Answer from the drawing. Dimensions are ordinates in mm from the lowest x, y and z of the part. A direction names the side the tool comes from. Coordinates: 2 decimals unless noted, no trailing zeros. Order: outer loops, then holes, each group sorted by start corner. A loop starts at its lowest first (then second) coordinate and runs counter-clockwise, first axis right, second up. Notation, with made-up numbers: (1, -27) -> (34, -27) arc R25 ccw to (34, -7) -> close; hole circle Ø4 at (-16.75, 20). An arc over 180 degrees is marked (long way). Answer as a JSON object with one key per item and string values. Group by question number.
1) Section D-D on y = 28 is taken. Determine the outline of the cut face in (x, z), and give its area (3 significant figures).
2) Determine the mould class of the marked faces 3, 4, 5 and 6 for opening direction X: released by +X, released by -X, zero draft, split by the parting line, or undercut.
3) Consider L1, parallel to Y at x = 43, z = 15.5; L2, parallel to X at y = 19.5, z = 13.75; L3, parallel to Z at x = 77.5, y = 32. Determine where each line is inside the solid, lowest interval first.
4) Section B-B on y = 4.5 is taken. Determine the outline of the cut face in (x, z).
5) Section A-A on x = 40 is taken. Determine the outline of the cut face in (y, z).
6) A tool of negligible diameter and unlimited length cuts with its end or side. For the marked faces 1 and 2, from which of +Z, -Z, +X, -X, +Y, -Y can it reach the whole face along a straight path? Write none if from no direction.
7) Section C-C on z = 5.25 is taken. Determine the outline of the cut face in (x, y), and give its area (3 significant figures).
8) Given pin 1 (2 mm diameter, centred on x = 70.5, z = 20.5, fed in from -Y), flat-ended and moving along its own axis, determine where the tip first touches the part or whether it passes through.
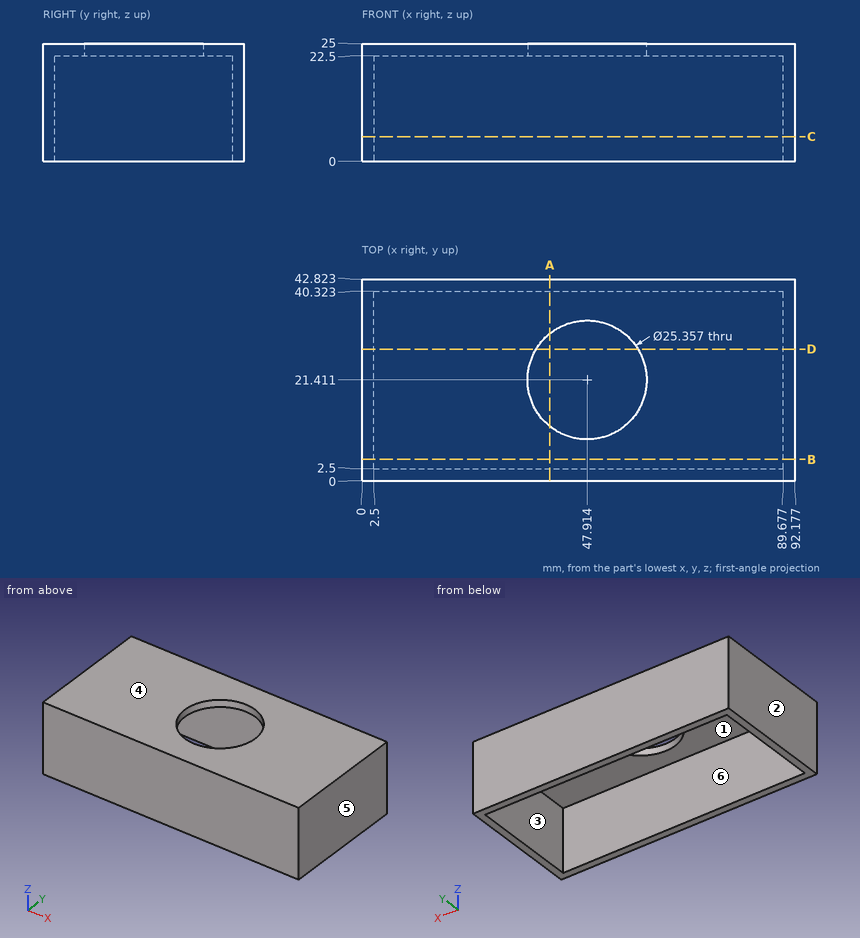
Worked answers:
{
 "1": {"outline": "(0, 0) -> (2.5, 0) -> (2.5, 22.5) -> (37.08, 22.5) -> (37.08, 25) -> (0, 25) -> close; (58.75, 22.5) -> (89.68, 22.5) -> (89.68, 0) -> (92.18, 0) -> (92.18, 25) -> (58.75, 25) -> close", "area": "289 mm²"},
 "2": {"face 3": "undercut", "face 4": "zero draft", "face 5": "released by +X", "face 6": "undercut"},
 "3": {"L1": "y = 0 to 2.5, 40.32 to 42.82", "L2": "x = 0 to 2.5, 89.68 to 92.18", "L3": "z = 22.5 to 25"},
 "4": {"outline": "(0, 0) -> (2.5, 0) -> (2.5, 22.5) -> (89.68, 22.5) -> (89.68, 0) -> (92.18, 0) -> (92.18, 25) -> (0, 25) -> close"},
 "5": {"outline": "(0, 0) -> (2.5, 0) -> (2.5, 22.5) -> (11.51, 22.5) -> (11.51, 25) -> (0, 25) -> close; (31.32, 22.5) -> (40.32, 22.5) -> (40.32, 0) -> (42.82, 0) -> (42.82, 25) -> (31.32, 25) -> close"},
 "6": {"face 1": "-Z", "face 2": "+Z, -Z, -X, +Y, -Y"},
 "7": {"outline": "(0, 0) -> (92.18, 0) -> (92.18, 42.82) -> (0, 42.82) -> close; hole (2.5, 2.5) -> (89.68, 2.5) -> (89.68, 40.32) -> (2.5, 40.32) -> close", "area": "650 mm²"},
 "8": {"pin 1": "stops at y = 0"}
}
